```python
from build123d import *

# Parameters (mm, degrees)
SKETCH_2_W          = 56
SKETCH_2_H          = 12
EXTRUDE_1_DEPTH     = 1.5
SKETCH_3_W          = 3
SKETCH_3_H          = 12
EXTRUDE_2_DEPTH     = 18
SKETCH_4_R          = 2.85
CUT_EXTRUDE_1_DEPTH = 54.077773126


with BuildPart() as part:
    # 草图2 → 凸台-拉伸1 (new body)
    with BuildSketch(Plane.XY):
        Rectangle(SKETCH_2_W, SKETCH_2_H)
    extrude(amount=EXTRUDE_1_DEPTH)

    # 草图3 → 凸台-拉伸2 (add)
    with BuildSketch(Plane.XY.offset(1.5)):
        with Locations((-20.5, 0)):
            Rectangle(SKETCH_3_W, SKETCH_3_H)
        with Locations((19.5, 0)):
            Rectangle(SKETCH_3_W, SKETCH_3_H)
    extrude(amount=EXTRUDE_2_DEPTH)

    # 草图4 → 切除-拉伸1 (cut, through all)
    with BuildSketch(Plane(origin=(21, 0, 0), x_dir=(0, 0, -1), z_dir=(1, 0, 0))):
        with Locations(Location((-13, 0, 0), (0, 0, 90))):
            Circle(SKETCH_4_R)
    extrude(amount=-CUT_EXTRUDE_1_DEPTH, mode=Mode.SUBTRACT)


solid = part.part
```
Read the model definition and answer for the solid it produces. Units are mm, in the model's axes. A direction names the side the tool comes from. Give positions to 0.01 mm unless a question says otherwise; leave off trailing zeros. Write each loop counter-clockwise with the first axis right and the second up, starting at its lowest first coordinate (ties: lowest second). Pieces come first, ordered by that corner, then holes. Notation, with made-up numbers: M -38.75,75.5 L 2.25,75.5 A17 cw 2.25,94.5 Z; hole C 71.25,45 d3. An arc over 180 degrees is marked long. Put each result on its own line as item: value. Start each with the question number.
1. Consider line 1 along Z through (x, y) = (-20.45, 0); line 2 along X through (y, z) = (-4.75, 14.75); line 3 along Z through (x, y) = (4, 1). Determine where each line is inside the solid, lowest interval first.
2. The part is cut by section A-A, the plane z = 7. Give the vertices of the cut face in (x, y), and give its area (3 significant figures).
3. The part is cut by section C-C, the plane z = 13. Give the vertices of the cut face in (x, y).
4. Each of these flat-tipped pins is pushed along its axis until it touches: pin 1 Ø1.5 at (x, y) = (11.5, 1) entering from +Z; pin 2 Ø6 at (y, z) = (1, 11.5) entering from +X; pin 3 Ø1 at (y, z) = (-2, 16.5) entering from -X; pin 4 Ø3 at (y, z) = (0.5, 13) entering from -X. Where does it stop, or does it pass through?
5. For a pull along Z with two mould halves and no side action, classify faces 1 (the flat face through (-28, 0, 1)), 2 (the flat face through (0, 0, 0)), 3 (the cylindrical face through (-20.479, -0.371, 15.826)) as released by +Z, released by -Z, zero draft, split by the parting line, or undercut.
6. Which of the six approach directions +Z, -Z, +X, -X, +Y, -Y give full straight-line access (tool end or side, diameter ignored) to faces 4 (the flat face through (-25, 0, 1.5)), 5 (the flat face through (-21, 0, 19.5)), 6 (the flat face through (21, 1, 10)), 7 (the flat face through (18, 1, 10))?
7. The part is cut by section D-D, the plane y = 3.5. Give the vertices of the cut face in (x, z).
8. The part is cut by section B-B, the plane y = 0.25. Give the vertices of the cut face in (x, z), and give its area (3 significant figures).
Final values:
1. line 1: z = 0 to 10.15, 15.85 to 19.5
1. line 2: x = -22 to -19, 18 to 21
1. line 3: z = 0 to 1.5
2. outline: M -22,-6 L -19,-6 L -19,6 L -22,6 Z; M 18,-6 L 21,-6 L 21,6 L 18,6 Z
2. area: 72.0 mm²
3. outline: M -22,-6 L -19,-6 L -19,-2.85 L -22,-2.85 Z; M -22,2.85 L -19,2.85 L -19,6 L -22,6 Z; M 18,-6 L 21,-6 L 21,-2.85 L 18,-2.85 Z; M 18,2.85 L 21,2.85 L 21,6 L 18,6 Z
4. pin 1: stops at z = 1.5
4. pin 2: stops at x = 21
4. pin 3: stops at x = -22
4. pin 4: passes through
5. face 1: zero draft
5. face 2: released by -Z
5. face 3: undercut
6. face 4: +Z, -X, +Y, -Y
6. face 5: +Z, +X, -X, +Y, -Y
6. face 6: +Z, +X, +Y, -Y
6. face 7: +Z, +Y, -Y
7. outline: M -28,0 L 28,0 L 28,1.5 L 21,1.5 L 21,19.5 L 18,19.5 L 18,1.5 L -19,1.5 L -19,19.5 L -22,19.5 L -22,1.5 L -28,1.5 Z
8. outline: M -28,0 L 28,0 L 28,1.5 L 21,1.5 L 21,10.16 L 18,10.16 L 18,1.5 L -19,1.5 L -19,10.16 L -22,10.16 L -22,1.5 L -28,1.5 Z; M -22,15.84 L -19,15.84 L -19,19.5 L -22,19.5 Z; M 18,15.84 L 21,15.84 L 21,19.5 L 18,19.5 Z
8. area: 158 mm²
